Read the model definition and answer for the solid it produces. Units are mm, in the model's axes. Face numbers are marked on the shaded views. Give positions to 0.01 mm unless a question says otherwise; leave off trailing zeros. Write each loop counter-clockwise with the first axis right and the second up, starting at its lowest first coordinate (ties: lowest second). Pieces come first, ordered by that corner, then holes. Notation, with made-up numbers: M 69,30 L 110,30 A28 ccw 110,63 Z; hole C 9.25,61 d4. An arc over 180 degrees is marked long. Put each result on its own line as item: value.
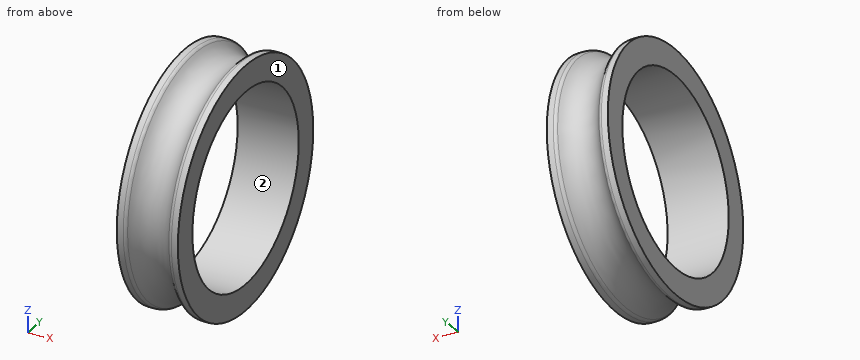
from build123d import *

# Parameters (mm, degrees)
F2_R = 0.5


with BuildPart() as f1:
    # F0 (on Top) → F1 (revolve)
    with BuildSketch(Plane.XY):
        with BuildLine():
            Line((-3.5, -1.5), (3.5, -1.5))
            Line((3.5, -1.5), (3.5, 1.5))
            Line((3.5, 1.5), (2.5, 1.5))
            ThreePointArc((2.5, 1.5), (0, 0.1583123952), (-2.5, 1.5))
            Line((-2.5, 1.5), (-3.5, 1.5))
            Line((-3.5, 1.5), (-3.5, -1.5))
        make_face()
    revolve(axis=Axis((0, -12.5, 0), (1, 0, 0)))

    # F2
    f2_edges = [f1.edges().sort_by_distance(p)[0] for p in [
        (-2.5, -26.5, 0),
        (2.5, -26.5, 0),
    ]]
    fillet(f2_edges, radius=F2_R)


solid = f1.part
(1) Section B-B on x = 1.25 is taken. Determine the outline of the cut face in (y, z).
Result:
outline: C -12.5,0 d25.86; hole C -12.5,0 d22
(2) Straight lines are drawn through the part: line 1 along Z through (x, y) = (2, -12.5); line 2 along Z through (x, y) = (-0.5, -6); line 3 along Y through (x, z) = (2.75, 3). For each, find the intervals that lie inside material, in ascending order. Write a range as from..to.
Result:
line 1: z = -13.42..-11, 11..13.42
line 2: z = -10.91..-8.87, 8.87..10.91
line 3: y = -26.17..-23.08, -1.92..1.17
(3) Section A-A on x = -0.25 is taken. Determine the outline of the cut face in (y, z).
Result:
outline: C -12.5,0 d25.34; hole C -12.5,0 d22
(4) Given pin 1 Ø2 at (x, y) = (2, -5) entering from -Z; pin 2 Ø3 at (x, z) = (2.5, -5) entering from -Y; pin 3 Ø1 at (x, z) = (2.5, -1.5) entering from +Y; pin 4 Ø12 at (y, z) = (-15.5, -5) entering from +X, each flat-ended and moving along its own axis, determine where each tip first touches the part or whether it passes through.
Result:
pin 1: stops at z = -12.26
pin 2: stops at y = -26.05
pin 3: stops at y = 1.46
pin 4: stops at x = 3.5
(5) For a pull along Z with two mould halves and no side action, classify the marked faces 1 and 2 as +Z half, -Z half, draft (parallel to the pull), parting line (faces both ways), or undercut.
Result:
face 1: draft
face 2: undercut
